Autodesk Inventor part; units mm, degrees
ref_plane "YZ Plane" through (0, 0, 0) normal (1, 0, 0) x (0, 1, 0)
ref_plane "XZ Plane" through (0, 0, 0) normal (0, 1, 0) x (-1, 0, 0)
ref_plane "XY Plane" through (0, 0, 0) normal (0, 0, 1) x (1, 0, 0)
sketch "Sketch1" plane through (0, 0, 0) normal (0, 0, 1) x (1, 0, 0)
  line L0 (0, 0) -> (25.4, 0)
  line L1 (25.4, 0) -> (25.4, 25.4)
  line L2 (25.4, 25.4) -> (0, 25.4)
  line L3 (0, 25.4) -> (0, 0)
  line L4 (1.5875, 23.8125) -> (23.8125, 23.8125)
  line L5 (23.8125, 23.8125) -> (23.8125, 1.5875)
  line L6 (23.8125, 1.5875) -> (1.5875, 1.5875)
  line L7 (1.5875, 1.5875) -> (1.5875, 23.8125)
  dimension "d0" = 25.4
  dimension "d1" = 25.4
  dimension "d2" = 1.5875
  dimension "d3" = 1.5875
  dimension "d4" = 1.5875
  dimension "d5" = 1.5875
extrude "Extrusion1" add sketch "Sketch1" along normal blind 762
sketch "Sketch2" plane through (25.4, 0, 0) normal (1, 0, 0) x (0, 0, -1)
  line L0 (0, 1.5875) -> (0, 23.8125)
  line L1 (0, 12.7) -> (-762, 12.7)
  line L2 (-762, 23.8125) -> (-762, 1.5875)
  line L3 (-762, 12.7) -> (-749.3, 12.7)
  line L4 (-749.3, 12.7) -> (-723.9, 12.7)
  line L5 (0, 12.7) -> (-12.7, 12.7)
  line L6 (-12.7, 12.7) -> (-38.1, 12.7)
  circle A0 centre (-12.7, 12.7) radius 2.54
  circle A1 centre (-38.1, 12.7) radius 2.54
  circle A2 centre (-723.9, 12.7) radius 2.54
  circle A3 centre (-749.3, 12.7) radius 2.54
  point P0 (0, 0)
  dimension "d8" = 12.7
  dimension "d9" = 25.4
  dimension "d10" = 12.7
  dimension "d11" = 25.4
  dimension "d12" = 5.08
extrude "Extrusion2" cut sketch "Sketch2" against normal blind 25.4
sketch "Sketch3" plane through (0, 25.4, 0) normal (0, 1, 0) x (1, 0, 0)
  line L0 (23.8125, 0) -> (1.5875, 0)
  line L1 (12.7, 0) -> (12.7, -762)
  line L2 (25.4, -762) -> (0, -762)
  line L3 (12.7, -762) -> (12.7, -749.3)
  line L4 (12.7, -749.3) -> (12.7, -723.9)
  line L5 (12.7, 0) -> (12.7, -12.7)
  line L6 (12.7, -12.7) -> (12.7, -38.1)
  circle A0 centre (12.7, -12.7) radius 2.54
  circle A1 centre (12.7, -38.1) radius 2.54
  circle A2 centre (12.7, -723.9) radius 2.54
  circle A3 centre (12.7, -749.3) radius 2.54
  point P0 (0, 0)
  dimension "d15" = 12.7
  dimension "d16" = 25.4
  dimension "d17" = 12.7
  dimension "d18" = 25.4
  dimension "d19" = 5.08
extrude "Extrusion3" cut sketch "Sketch3" against normal blind 25.4
properties part number "1x1" material "Aluminum 6061"
Source: CAD feature listing. Evaluate the final solid. Frame: model axes, mm. A direction names the side the tool comes from. Give positions to 0.01 mm unless a question says otherwise; leave off trailing zeros. Loops run counter-clockwise (first coordinate to the right, second up) from the corner with the lowest first, then second, coordinate; pieces in that order, holes last. Notation, with made-up numbers: (38.5, -39) -> (70.5, -39) arc R12 ccw to (70.5, -32) -> close; hole circle Ø4 at (67.25, 54). An arc over 180 degrees is marked (long way). Use a Markdown table: item, result. Add a question column.
1) Pull-direction query (X, two-part tool) for faces 3 (the face through (25.4, 13, 376)), 4 (the face through (13, 0, 376)), 5 (the face through (23.812, 13, 376)), 6 (the face through (0, 13, 376)); classes: +X half, -X half, draft (parallel to the pull), parting line (faces both ways), or undercut.
2) First-contact query: pin 1 (6 mm diameter, centred on y = 12.7, z = 749.3, fed in from +X); pin 2 (3 mm diameter, centred on x = 12.7, z = 749.3, fed in from -Y). Flat tips, straight axial feed; report the tip coordinate or a pass-through.
3) Section query A-A, the plane z = 216. Return the cut outline in (x, y), then the cut area to 3 significant figures.
4) Reachability of faces 1 (the face through (13, 25.4, 376)), 2 (the face through (1.588, 13, 376)) from +Z, -Z, +X, -X, +Y, -Y: full face, straight path, thin tool, end or side. Return the list, or none.
5) Line query: line 1 along Z through (x, y) = (12.7, 0.7); line 2 along X through (y, z) = (14, 678.5). Output: solid intervals per line, ascending. Write a range as [from, to].
Numbers:
| question | item | result |
|---|---|---|
| 1 | face 3 | +X half |
| 1 | face 4 | draft |
| 1 | face 5 | undercut |
| 1 | face 6 | -X half |
| 2 | pin 1 | stops at x = 25.4 |
| 2 | pin 2 | passes through |
| 3 | outline | (0, 0) -> (25.4, 0) -> (25.4, 25.4) -> (0, 25.4) -> close; hole (1.59, 1.59) -> (23.81, 1.59) -> (23.81, 23.81) -> (1.59, 23.81) -> close |
| 3 | area | 151 mm2 |
| 4 | face 1 | +Z, -Z, +X, -X, +Y |
| 4 | face 2 | +Z, -Z |
| 5 | line 1 | z = [0, 10.16], [15.24, 35.56], [40.64, 721.36], [726.44, 746.76], [751.84, 762] |
| 5 | line 2 | x = [0, 1.59], [23.81, 25.4] |
